Answer from the drawing. Dimensions are ordinates in mm from the lowest x, y and z of the part. Coordinates: 2 decimals unless noted, no trailing zeros. Order: outer loops, then holes, each group sorted by start corner. A loop starts at its lowest first (then second) coordinate and runs counter-clockwise, first axis right, second up. Notation, with made-up numbers: (20, 85.25) - (29, 85.25) arc R14 ccw to (29, 110.25) - close; hole circle Ø1 at (-35.5, -34.75). An arc over 180 degrees is marked (long way). Use CSV: the item, a comma, the result in double quotes. Start each with the question number.
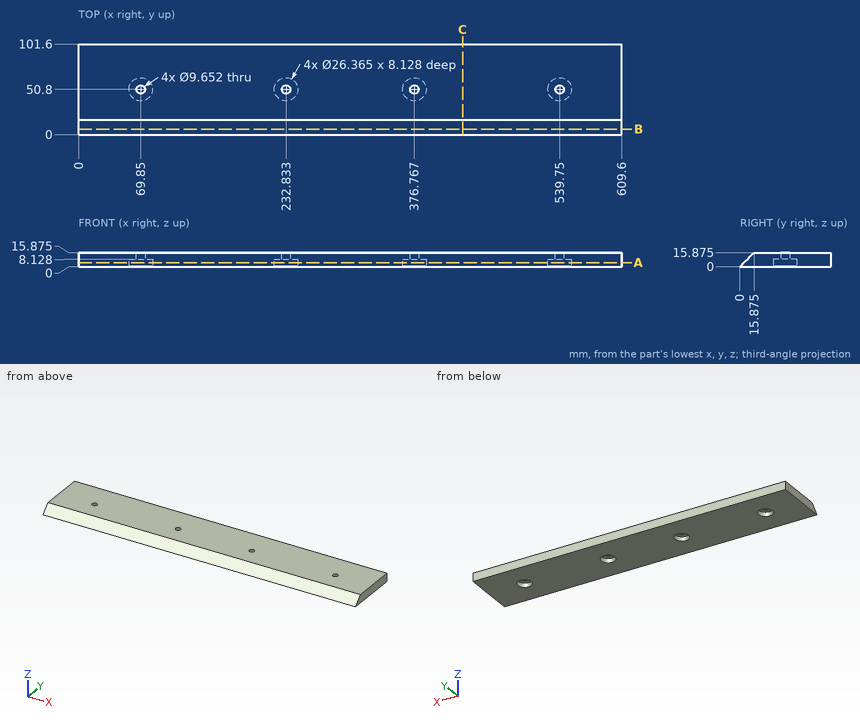
1) The part is cut by section B-B on y = 6. Determine the outline of the cut face in (x, z).
2) The part is cut by section C-C on x = 431. Determine the outline of the cut face in (y, z) (1 decimal).
3) The part is cut by section A-A on z = 4.5. State how many separate pieces and enclosed holes the cut face has, plus the area to 3 significant figures.
4) Flat-ended cylindrical pins translate along their axes: P1, Ø21, axis at x = 66, y = 56, coming from the -Z side; P2, Ø3, axis at x = 262.5, z = 3, coming from the -Y side; P3, Ø13, axis at x = 546, y = 52.5, coming from the -Z side. Find the tip coordinate at first contact, or state that the pin passes through.
5) Straight lines are drawn through the part: line 1 (X direction, y = 39.5, z = 5) (1 decimal); line 2 (X direction, y = 47, z = 2); line 3 (Y direction, x = 539.75, z = 13.5) (1 decimal). For each, find the intervals that lie inside material, in ascending order. Write a range as [from, to].
Answer key:
1,outline,"(0, 0) - (609.6, 0) - (609.6, 6) - (0, 6) - close"
2,outline,"(0, 0) - (101.6, 0) - (101.6, 15.9) - (15.9, 15.9) - close"
3,separate pieces,"1"
3,enclosed holes,"4"
3,area,"57,000 mm^2"
4,P1,"z = 0"
4,P2,"y = 1.5"
4,P3,"z = 8.13"
5,line 1,"[0, 63.1], [76.6, 226], [239.6, 370], [383.6, 533], [546.5, 609.6]"
5,line 2,"[0, 57.23], [82.47, 220.21], [245.46, 364.14], [389.39, 527.13], [552.37, 609.6]"
5,line 3,"[13.5, 46], [55.6, 101.6]"
